from build123d import *

# Parameters (mm, degrees)
F0_R     = 4.7625
F1_DEPTH = 50.8
F3_DEPTH = 6.35


with BuildPart() as f1:
    # F0 (on Right) → F1 (new body)
    with BuildSketch(Plane.YZ):
        Circle(F0_R)
    extrude(amount=F1_DEPTH)

    # F2 (on face) → F3 (join)
    with BuildSketch(Plane.YZ.offset(50.8)):
        Polygon((4.582718, 7.9375), (-4.582718, 7.9375), (-9.165436, 0), (-4.582718, -7.9375), (4.582718, -7.9375), (9.165436, 0), align=None)
    extrude(amount=F3_DEPTH)


solid = f1.part
Could you check a few things on this model? Use its own coordinates, in mm. A direction names the side the tool comes from. Give positions to 0.01 mm unless a question says otherwise; leave off trailing zeros. Order: outer loops, then holes, each group sorted by start corner. A loop starts at its lowest first (then second) coordinate and runs counter-clockwise, first axis right, second up.
1. Which directions (+Z, -Z, +X, -X, +Y, -Y) give clear straight access to the entire face, cutting with the end or side of a thin tool? Please do faces 1 (the flat face through (53.93, -6.91, -3.91)), 2 (the flat face through (50.8, 4, 4)).
Answers below:
face 1: -Z, +X, -X, -Y
face 2: -X
2. For pin 1 (8 mm diameter, centred on y = 4.5, z = 0.5, fed in from -X); pin 2 (5 mm diameter, centred on x = 25.5, z = 0, fed in from -Y); pin 3 (3 mm diameter, centred on x = 27.5, z = 4.5, fed in from -Y); pin 4 (1 mm diameter, centred on x = 46.5, z = 1, fed in from -Y), each with a flat end and sliding along its axis, tell me the tip position at first contact or that it passes through.
Answers below:
pin 1: stops at x = 0
pin 2: stops at y = -4.76
pin 3: stops at y = -3.7
pin 4: stops at y = -4.74
3. Suppose I cut it at D-D (y = -5.5). Write out the boundary of the cut face in (x, z).
Answers below:
outline: (50.8, -6.35) - (57.15, -6.35) - (57.15, 6.35) - (50.8, 6.35) - close
4. Suppose I cut it at A-A (y = 0). Write out the boundary of the cut face in (x, z).
Answers below:
outline: (0, -4.76) - (50.8, -4.76) - (50.8, -7.94) - (57.15, -7.94) - (57.15, 7.94) - (50.8, 7.94) - (50.8, 4.76) - (0, 4.76) - close
5. Suppose I cut it at C-C (x = 18). Write out the boundary of the cut face in (y, z) (1 decimal), plus the area to 3 significant figures.
Answers below:
outline: circle Ø9.5 at (0, 0)
area: 71.3 mm2
6. Suppose I cut it at B-B (z = -3). Write out the boundary of the cut face in (x, y).
Answers below:
outline: (0, -3.7) - (50.8, -3.7) - (50.8, -7.43) - (57.15, -7.43) - (57.15, 7.43) - (50.8, 7.43) - (50.8, 3.7) - (0, 3.7) - close
7. I need wall thicknesses on L1, parallel to Z at x = 21, y = -0.25; L2, parallel to X at y = 4.5, z = 6.5; L3, parallel to Z at x = 7.5, y = -1.25. Which ranges of each line are inside material? Lowest first, please.
Answers below:
L1: z = -4.76 to 4.76
L2: x = 50.8 to 57.15
L3: z = -4.6 to 4.6
